from build123d import *

# Parameters (mm, degrees)
SKETCH_1_R          = 2.15
SKETCH_1_R_2        = 7.125
EXTRUDE_1_DEPTH     = 5
SKETCH_2_R          = 4.5
CUT_EXTRUDE_1_DEPTH = 3
FILLET_1_R          = 1
CUT_EXTRUDE_2_DEPTH = 2
FILLET_2_R          = 1


with BuildPart() as part:
    # 草图1 → 凸台-拉伸1 (new body)
    with BuildSketch(Plane(origin=(0, 0, 0), x_dir=(0, 0, -1), z_dir=(1, 0, 0))):
        with BuildLine():
            Line((-23.090909091, -3.848365543), (-2.727272727, -9.620913858))
            ThreePointArc((-2.727272727, -9.620913858), (4.253098654, -9.050477989), (9.147283393, -4.040693817))
            Line((9.147283393, -4.040693817), (13.573641697, 5.979653091))
            ThreePointArc((13.573641697, 5.979653091), (13.638118854, 9.867579581), (10.897437667, 12.625984252))
            Line((10.897437667, 12.625984252), (1.979480632, 16.283858268))
            ThreePointArc((1.979480632, 16.283858268), (-9.5, 33.4), (1.979480632, 50.516141732))
            Line((1.979480632, 50.516141732), (10.897437667, 54.174015748))
            ThreePointArc((10.897437667, 54.174015748), (13.545928712, 60.881953925), (6.736898846, 63.258516924))
            Line((6.736898846, 63.258516924), (-8.810480924, 55.366813539))
            ThreePointArc((-8.810480924, 55.366813539), (-10.081211961, 54.350712224), (-10.842152772, 52.912592502))
            Line((-10.842152772, 52.912592502), (-25.842152772, 1.112592502))
            ThreePointArc((-25.842152772, 1.112592502), (-25.498078189, -1.939961078), (-23.090909091, -3.848365543))
        make_face()
        with Locations((9, 58.8)):
            Circle(SKETCH_1_R, mode=Mode.SUBTRACT)
        with Locations((-22, 0)):
            Circle(SKETCH_1_R, mode=Mode.SUBTRACT)
        with Locations((-7, 51.8)):
            Circle(SKETCH_1_R, mode=Mode.SUBTRACT)
        with Locations((9, 8)):
            Circle(SKETCH_1_R, mode=Mode.SUBTRACT)
        Circle(SKETCH_1_R_2, mode=Mode.SUBTRACT)
    extrude(amount=EXTRUDE_1_DEPTH)

    # 草图2 → 切除-拉伸1 (cut)
    with BuildSketch(Plane.ZY):
        with Locations((22, 0)):
            Circle(SKETCH_2_R)
    extrude(amount=-CUT_EXTRUDE_1_DEPTH, mode=Mode.SUBTRACT)

    # 圆角1
    fillet_1_edges = [part.edges().sort_by_distance(p)[0] for p in [
        (1.5, 3.092792715, 25.268735722),
        (1.5, -4.41060722, 21.107506888),
    ]]
    fillet(fillet_1_edges, radius=FILLET_1_R)

    # 草图3 → 切除-拉伸2 (cut)
    with BuildSketch(Plane.ZY):
        with BuildLine():
            Line((-3.75, 58.8), (-3.75, 51.242354784))
            Line((-3.75, 51.242354784), (-9.416400073, 53.566539292))
            ThreePointArc((-9.416400073, 53.566539292), (-12.562049945, 62.65672143), (-3.75, 58.8))
        make_face()
        with BuildLine():
            Line((-3.75, 8), (-3.75, 15.557645216))
            Line((-3.75, 15.557645216), (-9.416400073, 13.233460708))
            ThreePointArc((-9.416400073, 13.233460708), (-12.562049945, 4.14327857), (-3.75, 8))
        make_face()
    extrude(amount=-CUT_EXTRUDE_2_DEPTH, mode=Mode.SUBTRACT)

    # 圆角2
    fillet_2_edges = [part.edges().sort_by_distance(p)[0] for p in [
        (1, 5.693326891, -4.283883041),
        (1, 3.586845523, -6.156310924),
        (1, 62.533971032, -5.309476957),
        (1, 4.515373291, -12.926815084),
        (1, 15.557645216, -3.75),
        (1, 51.242354784, -3.75),
    ]]
    fillet(fillet_2_edges, radius=FILLET_2_R)


solid = part.part
Read the model definition and answer for the solid it produces. Units are mm, in the model's axes. A direction names the side the tool comes from. Give positions to 0.01 mm unless a question says otherwise; leave off trailing zeros. Write each loop counter-clockwise with the first axis right and the second up, starting at its lowest first coordinate (ties: lowest second). Pieces come first, ordered by that corner, then holes. Notation, with made-up numbers: (55.5, 5) - (110.5, 5) arc R36 ccw to (110.5, 42) - close; hole circle Ø8 at (32, 65.25). An arc over 180 degrees is marked (long way). Return JSON: item names as keys, results as strings.
Q1. For faces 4 (the face through (1.479, -4.377, 19.356)), 5 (the face through (1.48, 2.26, 18.11)), 6 (the face through (2.465, 27.375, 18.237)), 7 (the face through (3.58, 14.43, -6.5)), determine the directions among +Z, -Z, +X, -X, +Y, -Y from which every point of the face is accessible in a straight line to the end or side of a thin tool.
Reply:
{"face 4": "+Z, -X", "face 5": "-X", "face 6": "+Z, +X, -X, +Y", "face 7": "-Z, +X, -X"}
Q2. Consider line 1 along Y through (x, z) = (1.8, 8); line 2 along Y through (x, z) = (2.8, -9); line 3 along Y through (x, z) = (4.7, 4). Determine where each line is inside the solid, lowest interval first. Write a range as [from, to].
Reply:
{"line 1": "[-8.13, 26.1], [40.7, 49.9], [53.7, 55.78]", "line 2": "[-4.36, 5.85], [10.15, 13.4], [53.4, 56.65], [60.95, 63.8]", "line 3": "[-9.26, -5.9], [5.9, 20.24], [46.56, 57.81]"}
Q3. A cutting plane is placed at A-A, the plane z = 22. Determine the outline of the cut face in (x, y).
Reply:
{"outline": "(0, 4.5) - (3, 4.5) - (3, 2.15) - (5, 2.15) - (5, 14.38) - (0, 14.38) - close; (3, -4.16) - (5, -4.16) - (5, -2.15) - (3, -2.15) - close"}
Q4. A cutting plane is placed at B-B, the plane z = 0. Determine the outline of the cut face in (x, y) (3 decimals), and give its area (3 significant figures).
Reply:
{"outline": "(0, -10) - (5, -10) - (5, -7.125) - (0, -7.125) - close; (0, 7.125) - (5, 7.125) - (5, 17.237) - (0, 17.237) - close; (0, 49.563) - (5, 49.563) - (5, 59.839) - (0, 59.839) - close", "area": "116 mm²"}
Q5. Given P1, Ø6, axis at y = 37, z = 11.5, coming from the -X side; P2, Ø2.5, axis at y = 58.8, z = -9, coming from the +X side; P3, Ø0.6, axis at x = 1.5, y = 12.5, coming from the -Z side; P4, Ø5, axis at y = 0, z = 22, coming from the -X side, each flat-ended and moving along its own axis, determine where each tip first touches the part or whether it passes through.
Reply:
{"P1": "x = 0", "P2": "through", "P3": "z = -3.75", "P4": "x = 3"}
Q6. For a pull along Z with two mould halves and no side action, classify faces 1 (the face through (2.465, -6.694, 13.052)), 2 (the face through (5, 19, 6)), 3 (the face through (0.99, 2.76, -9.29)) as released by +Z, released by -Z, zero draft, split by the parting line, or undercut.
Reply:
{"face 1": "released by +Z", "face 2": "zero draft", "face 3": "undercut"}
Q7. A cutting plane is placed at C-C, the plane y = 26. Determine the outline of the cut face in (x, z), and give its area (3 significant figures).
Reply:
{"outline": "(0, 7.96) - (5, 7.96) - (5, 18.64) - (0, 18.64) - close", "area": "53.4 mm²"}
